Autodesk Inventor part; units mm, degrees
ref_plane "Work Plane1" through (0, 0, 0) normal (1, 0, 0) x (0, 1, 0)
ref_plane "XZ Plane" through (0, 0, 0) normal (0, 1, 0) x (-1, 0, 0)
ref_plane "XY Plane" through (0, 0, 0) normal (0, 0, 1) x (1, 0, 0)
sketch "Sketch1" plane through (0, 0, 0) normal (0, 0, 1) x (1, 0, 0)
  line L0 (2.3094, 4) -> (4.6188, 0)
  line L1 (4.6188, 0) -> (2.3094, -4)
  line L2 (2.3094, -4) -> (-2.3094, -4)
  line L3 (-2.3094, -4) -> (-4.6188, 0)
  line L4 (-4.6188, 0) -> (-2.3094, 4)
  line L5 (-2.3094, 4) -> (2.3094, 4)
  point P0 (0, 0)
  point P1 (0, 0)
  dimension "d0" = 8
extrude "Extrusion1" add sketch "Sketch1" along normal blind 3
ref_plane "Work Plane1" through (0, 0, 0) normal (1, 0, 0) x (0, 1, 0)
sketch "Sketch2" plane through (0, 0, 0) normal (1, 0, 0) x (0, 1, 0)
  line L0 (0, 0) -> (-4, 0)
  line L1 (0, 0) -> (0, 3)
  line L2 (-4, 3) -> (0, 3)
  line L3 (-4, 0) -> (-4, 3)
  line L4 (4, 0) -> (0, 0)
  line L5 (4, 0) -> (4, 3)
  line L6 (0, 3) -> (4, 3)
  line L7 (0, 0) -> (0, 3)
  line L8 (0, 3) -> (0, 5)
  line L9 (0, 5) -> (0.75, 5)
  line L10 (0.75, 5) -> (2.75, 3)
  line L11 (0, 3) -> (2.75, 3)
  point P0 (0, 0)
  dimension "d4" = 2
  dimension "d5" = 0.75
  dimension "d6" = 2.75
revolve "Revolution1" add sketch "Sketch2" angle 360 about axis through (0, 0, 3) along (0, 0, 1) contours L8 L9 L10 L6
sketch "Sketch3" plane through (0, 0, 5) normal (0, 0, 1) x (1, 0, 0)
  circle A0 centre (0, 0) radius 0.75
  circle A1 centre (0, 0) radius 0.2
  dimension "d8" = 0.4
extrude "Extrusion2" cut sketch "Sketch3" against normal through all contours A1
properties part number "nozzle" material "Brass, Soft Yellow"
Verification items for the finished model (mm, model axes). A direction names the side the tool comes from. Coordinates: 2 decimals unless noted, no trailing zeros. Loops run counter-clockwise (first coordinate to the right, second up) from the corner with the lowest first, then second, coordinate; pieces in that order, holes last. Notation, with made-up numbers: (12.5, 52.25) - (65.5, 52.25) arc R21 ccw to (65.5, 91.25) - close; hole circle Ø7 at (-22.75, -36). An arc over 180 degrees is marked (long way). Answer as a JSON object with one key per item and string values.
(1) Access from +Z, -Z, +X, -X, +Y, -Y to the whole of each face (thin tool, end or side, straight path). Record for faces 1 (the flat face through (1, 3, 3)), 2 (the flat face through (-3.48, 1.97, 1.48)).
Response:
{"face 1": "+Z", "face 2": "+Z, -Z, -X, +Y"}
(2) Cross-section at C-C, the plane z = 3.65. Record the boundary of the cut face in (x, y), then the cut area to 3 significant figures.
Response:
{"outline": "circle Ø4.2 at (0, 0); hole circle Ø0.4 at (0, 0)", "area": "13.7 mm²"}
(3) Cross-section at B-B, the plane z = 1.35. Record the boundary of the cut face in (x, y).
Response:
{"outline": "(-4.62, 0) - (-2.31, -4) - (2.31, -4) - (4.62, 0) - (2.31, 4) - (-2.31, 4) - close; hole circle Ø0.4 at (0, 0)"}
(4) Go/stop test with a flat-tipped pin: pin 1 Ø3 at (x, y) = (-2, 0) entering from +Z. Record where the tip stops, or that it passes through.
Response:
{"pin 1": "stops at z = 5"}
(5) Cross-section at A-A, the plane x = 0. Record the boundary of the cut face in (y, z), then the cut area to 3 significant figures.
Response:
{"outline": "(-4, 0) - (-0.2, 0) - (-0.2, 5) - (-0.75, 5) - (-2.75, 3) - (-4, 3) - close; (0.2, 0) - (4, 0) - (4, 3) - (2.75, 3) - (0.75, 5) - (0.2, 5) - close", "area": "29.0 mm²"}
(6) Scan lines: line 1 along Y through (x, z) = (0, 2.25); line 2 along Z through (x, y) = (2, -2.5); line 3 along Z through (x, y) = (2, -0.5). Record each from-to range of solid material in increasing order.
Response:
{"line 1": "y = -4 to -0.2, 0.2 to 4", "line 2": "z = 0 to 3", "line 3": "z = 0 to 3.69"}
(7) Cross-section at D-D, the plane y = 3. Record the boundary of the cut face in (x, z).
Response:
{"outline": "(-2.89, 0) - (2.89, 0) - (2.89, 3) - (-2.89, 3) - close"}
